```python
from build123d import *

# Parameters (mm, degrees)
EXTRUDE_1_DEPTH     = 1000
CUT_EXTRUDE_1_REACH = 1005.594
SKETCH_2_R          = 25


with BuildPart() as part:
    # 草图1 → 凸台-拉伸1 (new body)
    with BuildSketch(Plane.XY):
        with BuildLine():
            Line((-55, 30), (55, 30))
            ThreePointArc((55, 30), (58.535533906, 28.535533906), (60, 25))
            Line((60, 25), (60, -25))
            ThreePointArc((60, -25), (58.535533906, -28.535533906), (55, -30))
            Line((55, -30), (-55, -30))
            ThreePointArc((-55, -30), (-58.535533906, -28.535533906), (-60, -25))
            Line((-60, -25), (-60, 25))
            ThreePointArc((-60, 25), (-58.535533906, 28.535533906), (-55, 30))
        make_face()
        with BuildLine():
            Line((-55, 26), (55, 26))
            ThreePointArc((55, 26), (55.707106781, 25.707106781), (56, 25))
            Line((56, 25), (56, -25))
            ThreePointArc((56, -25), (55.707106781, -25.707106781), (55, -26))
            Line((55, -26), (-55, -26))
            ThreePointArc((-55, -26), (-55.707106781, -25.707106781), (-56, -25))
            Line((-56, -25), (-56, 25))
            ThreePointArc((-56, 25), (-55.707106781, 25.707106781), (-55, 26))
        make_face(mode=Mode.SUBTRACT)
    extrude(amount=EXTRUDE_1_DEPTH)

    # 草图2 → 切除-拉伸1 (cut, up to next)
    with BuildSketch(Plane.XZ.offset(30), mode=Mode.PRIVATE) as cut_extrude_1_sk1:
        with Locations(Location((0, 960, 0), (0, 0, 270))):
            Circle(SKETCH_2_R)
    cut_extrude_1_tool1 = extrude(cut_extrude_1_sk1.sketch, amount=-CUT_EXTRUDE_1_REACH, mode=Mode.PRIVATE) & part.part
    add(cut_extrude_1_tool1.solids().sort_by_distance((0, -30, 960))[0], mode=Mode.SUBTRACT)


solid = part.part
```
Check sheet for the modelled part. Datum: model origin and axes. Units: mm. A direction names the side the tool comes from. Give positions to 0.01 mm unless a question says otherwise; leave off trailing zeros. Loops run counter-clockwise (first coordinate to the right, second up) from the corner with the lowest first, then second, coordinate; pieces in that order, holes last. Notation, with made-up numbers: (-12, 45.5) - (13, 45.5) arc R33 cw to (13, 75.5) - close; hole circle Ø5 at (-27, 79.25). An arc over 180 degrees is marked (long way). One line per question, with ' | ' between items. Start each with the question number.
1. Cross-section at A-A, the plane x = 0. Enter the section's corners in (y, z).
2. Cross-section at B-B, the plane x = 38. Enter the section's corners in (y, z), plus the area to 3 significant figures.
3. Cross-section at D-D, the plane z = 380. Enter the section's corners in (x, y).
4. Set-up check for faces 1 (the flat face through (-1, 30, 493)), 2 (the flat face through (-56, 0, 493)): record each of +Z, -Z, +X, -X, +Y, -Y from which the full face is reachable in a straight line by a thin tool's end or side.
5. Material ranges on line 1 along X through (y, z) = (10, 269.5); line 2 along Y through (x, z) = (37, 666); line 3 along X through (y, z) = (-28.25, 960), recorded low to high. Write a range as [from, to].
6. Cross-section at C-C, the plane y = 6. Enter the section's corners in (x, z).
7. Draft check along Y on faces 3 (the flat face through (1, -30, 493)), 4 (the cylindrical face through (1.099, -28.028, 984.976)), 5 (the flat face through (56, 0, 493)). Enter one of: released by +Y, released by -Y, zero draft, split by the parting line, or undercut.
Check result:
1) outline: (-30, 0) - (-26, 0) - (-26, 935) - (-30, 935) - close; (-30, 985) - (-26, 985) - (-26, 1000) - (-30, 1000) - close; (26, 0) - (30, 0) - (30, 1000) - (26, 1000) - close
2) outline: (-30, 0) - (-26, 0) - (-26, 1000) - (-30, 1000) - close; (26, 0) - (30, 0) - (30, 1000) - (26, 1000) - close | area: 8,000 mm2
3) outline: (-60, -25) arc R5 ccw to (-55, -30) - (55, -30) arc R5 ccw to (60, -25) - (60, 25) arc R5 ccw to (55, 30) - (-55, 30) arc R5 ccw to (-60, 25) - close; hole (-56, -25) arc R1 ccw to (-55, -26) - (55, -26) arc R1 ccw to (56, -25) - (56, 25) arc R1 ccw to (55, 26) - (-55, 26) arc R1 ccw to (-56, 25) - close
4) face 1: +Z, -Z, +X, -X, +Y | face 2: +Z, -Z
5) line 1: x = [-60, -56], [56, 60] | line 2: y = [-30, -26], [26, 30] | line 3: x = [-58.8, -25], [25, 58.8]
6) outline: (-60, 0) - (-56, 0) - (-56, 1000) - (-60, 1000) - close; (56, 0) - (60, 0) - (60, 1000) - (56, 1000) - close
7) face 3: released by -Y | face 4: zero draft | face 5: undercut
